Could you check a few things on this model? Use its own coordinates, in mm. Round coordinates to 2 decimals unless told otherwise and drop trailing zeros. Order: outer loops, then holes, each group sorted by start corner. A loop starts at its lowest first (then second) coordinate and runs counter-clockwise, first axis right, second up. Notation, with made-up numbers: M 72.25,53 L 106.25,53 A11 cw 106.25,59 Z; hole C 28.5,28 d5. An arc over 180 degrees is marked long. Write each question's results on one line, items separated by ' | '. Start each with the question number.
1. Please list where these lines run through material, in increasing order: L1, parallel to X at y = 45, z = 0.5; L2, parallel to Y at x = -4.25, z = 8; L3, parallel to X at y = 14, z = -8.5.
2. Suppose I cut it at A-A on y = 9. Write out the boundary of the cut face in (x, z), and give its area (3 significant figures).
3. I'm going to push flat-ended pins straight in: pin 1 (4 mm diameter, centred on y = 36.5, z = 7, fed in from +X); pin 2 (2 mm diameter, centred on y = 21.5, z = 3, fed in from -X); pin 3 (10 mm diameter, centred on x = -6, z = -4.5, fed in from +Y). Where does each tip first touch, or does it pass through?
from build123d import *

# Parameters (mm, degrees)
SKETCH1_R           = 11
BOSS_EXTRUDE1_DEPTH = 65
SKETCH2_R           = 1.5
BOSS_EXTRUDE2_DEPTH = 9.5
FILLET1_R           = 1.3
FILLET2_R           = 8
FILLET3_R           = 2
FILLET4_R           = 2


with BuildPart() as part:
    # Sketch1 → Boss-Extrude1 (new body)
    with BuildSketch(Plane(origin=(0, 0, 0), x_dir=(1, 0, 0), z_dir=(0, 1, 0))):
        Circle(SKETCH1_R)
    extrude(amount=BOSS_EXTRUDE1_DEPTH)

    # Sketch2 → Boss-Extrude2 (add)
    with BuildSketch(Plane(origin=(0, 65, 0), x_dir=(1, 0, 0), z_dir=(0, 1, 0))):
        Circle(SKETCH2_R)
    extrude(amount=BOSS_EXTRUDE2_DEPTH)

    # Fillet1
    fillet1_edges = [part.edges().sort_by_distance(p)[0] for p in [
        (-1.5, 74.5, 0),
    ]]
    fillet(fillet1_edges, radius=FILLET1_R)

    # Fillet2
    fillet2_edges = [part.edges().sort_by_distance(p)[0] for p in [
        (-1.5, 65, 0),
    ]]
    fillet(fillet2_edges, radius=FILLET2_R)

    # Fillet3
    fillet3_edges = [part.edges().sort_by_distance(p)[0] for p in [
        (-11, 65, 0),
    ]]
    fillet(fillet3_edges, radius=FILLET3_R)

    # Fillet4
    fillet4_edges = [part.edges().sort_by_distance(p)[0] for p in [
        (-11, 0, 0),
    ]]
    fillet(fillet4_edges, radius=FILLET4_R)


solid = part.part
Filled sheet:
1) L1: x = -10.99 to 10.99 | L2: y = 0 to 65.01 | L3: x = -6.98 to 6.98
2) outline: C 0,0 d22 | area: 380 mm^2
3) pin 1: stops at x = 9.8 | pin 2: stops at x = -10.82 | pin 3: stops at y = 69.13
